For this review, take the finished solid that the model builds, in its own axes (mm). Face numbers are marked on the shaded views. A direction names the side the tool comes from. Coordinates: 2 decimals unless noted, no trailing zeros. Write each loop counter-clockwise with the first axis right and the second up, starting at its lowest first coordinate (ties: lowest second). Pieces come first, ordered by that corner, then holes. Notation, with made-up numbers: M -36,82.25 L -22,82.25 A21 ccw -22,115.25 Z; hole C -28,50 d4. An arc over 180 degrees is marked long. Return JSON: item names as keys, results as strings.
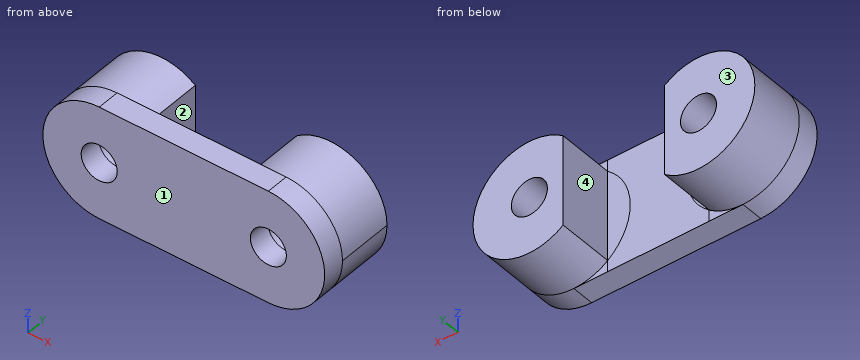
```python
from build123d import *

# Parameters (mm, degrees)
SKETCH1_R           = 1.6
BOSS_EXTRUDE1_DEPTH = 2
SKETCH2_R           = 5
SKETCH2_R_2         = 1.6
BOSS_EXTRUDE2_DEPTH = 5
SKETCH3_W           = 9
SKETCH3_H           = 5
CUT_EXTRUDE1_DEPTH  = 11


with BuildPart() as part:
    # Sketch1 → Boss-Extrude1 (new body)
    with BuildSketch(Plane(origin=(0, 0, 0), x_dir=(1, 0, 0), z_dir=(0, 1, 0))):
        with BuildLine():
            Line((-7.5, 5), (7.5, 5))
            ThreePointArc((7.5, 5), (12.5, 0), (7.5, -5))
            Line((7.5, -5), (-7.5, -5))
            ThreePointArc((-7.5, -5), (-12.5, 0), (-7.5, 5))
        make_face()
        with Locations((-7.5, 0)):
            Circle(SKETCH1_R, mode=Mode.SUBTRACT)
        with Locations((7.5, 0)):
            Circle(SKETCH1_R, mode=Mode.SUBTRACT)
    extrude(amount=BOSS_EXTRUDE1_DEPTH)

    # Sketch2 → Boss-Extrude2 (add)
    with BuildSketch(Plane(origin=(0, 2, 0), x_dir=(1, 0, 0), z_dir=(0, 1, 0))):
        with Locations((-7.5, 0)):
            Circle(SKETCH2_R)
        with Locations((-7.5, 0)):
            Circle(SKETCH2_R_2, mode=Mode.SUBTRACT)
        with Locations((7.5, 0)):
            Circle(SKETCH2_R)
        with Locations((7.5, 0)):
            Circle(SKETCH2_R_2, mode=Mode.SUBTRACT)
    extrude(amount=BOSS_EXTRUDE2_DEPTH)

    # Sketch3 → Cut-Extrude1 (cut, through all)
    with BuildSketch(Plane.XY.offset(5)):
        with Locations((0, 4.5)):
            Rectangle(SKETCH3_W, SKETCH3_H)
    extrude(amount=-CUT_EXTRUDE1_DEPTH, mode=Mode.SUBTRACT)


solid = part.part
```
1. We need section D-D (z = -3). State the section outline as (x, y) points, plus the area to 3 significant figures.
Checks:
{"outline": "M -11.5,0 L 11.5,0 L 11.5,7 L 4.5,7 L 4.5,2 L -4.5,2 L -4.5,7 L -11.5,7 Z", "area": "116 mm2"}
2. Clearance check with flat-ended pins moving along their axes: pin 1 Ø1.6 at (x, z) = (-3.5, 0.5) entering from +Y; pin 2 Ø1.5 at (y, z) = (4, -1.5) entering from -X; pin 3 Ø1 at (y, z) = (6, -1) entering from -X. State where each tip first meets the part, or that it passes through.
Checks:
{"pin 1": "y = 2", "pin 2": "x = -12.44", "pin 3": "x = -12.47"}
3. We need section A-A (y = 3.5). State the section outline as (x, z) points.
Checks:
{"outline": "M -4.5,-4 L -4.5,4 A5 ccw long Z; M 4.5,-4 A5 ccw long 4.5,4 Z; hole C -7.5,0 d3.2; hole C 7.5,0 d3.2"}
4. Wall thickness on L1, parallel to X at y = 5.2, z = 0; L2, parallel to X at y = 0.5, z = 0; L3, parallel to Z at x = -7.5, y = 3.7: over which ranges is each line inside the solid? List them lowest first. Write a range as from..to.
Checks:
{"L1": "-12.5..-9.1, -5.9..-4.5, 4.5..5.9, 9.1..12.5", "L2": "-12.5..-9.1, -5.9..5.9, 9.1..12.5", "L3": "-5..-1.6, 1.6..5"}
5. We need section B-B (z = -0.75). State the section outline as (x, y) points.
Checks:
{"outline": "M -12.44,0 L -8.91,0 L -8.91,7 L -12.44,7 Z; M -6.09,0 L 6.09,0 L 6.09,7 L 4.5,7 L 4.5,2 L -4.5,2 L -4.5,7 L -6.09,7 Z; M 8.91,0 L 12.44,0 L 12.44,7 L 8.91,7 Z"}
6. For the marked faces 3 and 4, list the 3-axis set-ups (+Z, -Z, +X, -X, +Y, -Y) from which the entire face can be reached by the end or side of a thin tool; tool diameter is ignored.
Checks:
{"face 3": "+Z, -Z, +X, -X, +Y", "face 4": "+Z, -Z, +Y"}
7. Draft analysis for pull direction X (two halves, no side actions). For the marked faces 1 and 2, state which applies: +X half, -X half, draft (parallel to the pull), parting line (faces both ways), or undercut.
Checks:
{"face 1": "draft", "face 2": "undercut"}
8. We need section C-C (x = 8.5). State the section outline as (y, z) points.
Checks:
{"outline": "M 0,-4.9 L 7,-4.9 L 7,-1.25 L 0,-1.25 Z; M 0,1.25 L 7,1.25 L 7,4.9 L 0,4.9 Z"}
